Can you work these out from the model? Positions are in its coordinate system, mm. A direction names the side the tool comes from. Give positions to 0.01 mm unless a question says otherwise; leave off trailing zeros. Write each loop counter-clockwise with the first axis right and the second up, starting at its lowest first coordinate (ties: lowest second). Pieces come first, ordered by that corner, then holes.
```python
from build123d import *

# Parameters (mm, degrees)
SKETCH1_R           = 6
SKETCH1_R_2         = 4
BOSS_EXTRUDE1_DEPTH = 10
SKETCH2_R           = 6
BOSS_EXTRUDE2_DEPTH = 8
SKETCH3_R           = 5
SKETCH3_R_2         = 3
BOSS_EXTRUDE3_DEPTH = 10
SKETCH4_R           = 1.5
CUT_EXTRUDE1_DEPTH  = 10
SKETCH5_W           = 1.364712806
SKETCH5_H           = 6.528107361
CUT_EXTRUDE2_DEPTH  = 10
CHAMFER1_SIZE       = 1
SKETCH6_W           = 0.953233667
SKETCH6_H           = 4.701860643
CUT_EXTRUDE3_DEPTH  = 10


with BuildPart() as part:
    # Sketch1 → Boss-Extrude1 (new body)
    with BuildSketch(Plane(origin=(0, 0, 0), x_dir=(1, 0, 0), z_dir=(0, 1, 0))):
        with Locations(Location((0, 0, 0), (0, 0, 270))):
            Circle(SKETCH1_R)
        with Locations(Location((0, 0, 0), (0, 0, 270))):
            Circle(SKETCH1_R_2, mode=Mode.SUBTRACT)
    extrude(amount=BOSS_EXTRUDE1_DEPTH)

    # Sketch2 → Boss-Extrude2 (add)
    with BuildSketch(Plane(origin=(0, 10, 0), x_dir=(1, 0, 0), z_dir=(0, 1, 0))):
        with Locations(Location((0, 0, 0), (0, 0, 270))):
            Circle(SKETCH2_R)
    extrude(amount=BOSS_EXTRUDE2_DEPTH)

    # Sketch3 → Boss-Extrude3 (add)
    with BuildSketch(Plane(origin=(0, 18, 0), x_dir=(1, 0, 0), z_dir=(0, 1, 0))):
        with Locations(Location((0, 0, 0), (0, 0, 270))):
            Circle(SKETCH3_R)
        with Locations(Location((0, 0, 0), (0, 0, 270))):
            Circle(SKETCH3_R_2, mode=Mode.SUBTRACT)
    extrude(amount=BOSS_EXTRUDE3_DEPTH)

    # Sketch4 → Cut-Extrude1 (cut)
    with BuildSketch(Plane(origin=(0, 0, 0), x_dir=(0, 0, -1), z_dir=(1, 0, 0))):
        with Locations(Location((0, 5, 0), (0, 0, 180))):
            Circle(SKETCH4_R)
        with Locations(Location((0, 23, 0), (0, 0, 180))):
            Circle(SKETCH4_R)
    extrude(amount=CUT_EXTRUDE1_DEPTH, mode=Mode.SUBTRACT)

    # Sketch5 → Cut-Extrude2 (cut)
    with BuildSketch(Plane.XZ):
        with Locations((6.382356403, -0.325289304)):
            Rectangle(SKETCH5_W, SKETCH5_H)
    extrude(amount=-CUT_EXTRUDE2_DEPTH, mode=Mode.SUBTRACT)

    # Chamfer1
    # the kernel refuses this chamfer: 1 mm, written as the material it adds along each edge
    with BuildSketch(Plane(origin=(5.7, 10, -4.445182387), x_dir=(-0.02749587661058651, -0.9996219169112968, 0), z_dir=(0, 0, 1))) as chamfer1_piece_1_section:
        Polygon((CHAMFER1_SIZE * 0.999621916911, CHAMFER1_SIZE * 0.0274958766106), (-CHAMFER1_SIZE * 0.0274958766106, CHAMFER1_SIZE * 0.999621916911), (0, 0), align=None)
    chamfer1_piece_1 = extrude(amount=8.890364775, mode=Mode.PRIVATE)
    chamfer1_piece_1 = chamfer1_piece_1 & Plane(origin=(0, 9.556619027, 0), x_dir=(0, 0, 1), z_dir=(0, -1, 0)) * Cylinder(6, 22, mode=Mode.PRIVATE)
    add(chamfer1_piece_1)

    # Sketch6 → Cut-Extrude3 (cut)
    with BuildSketch(Plane(origin=(0, 28, 0), x_dir=(1, 0, 0), z_dir=(0, 1, 0))):
        with Locations((5.176616834, 0.047714229)):
            Rectangle(SKETCH6_W, SKETCH6_H)
    extrude(amount=-CUT_EXTRUDE3_DEPTH, mode=Mode.SUBTRACT)


solid = part.part
```
1) Please list where these lines run through material, in increasing order: L1, parallel to Y at x = 4.15, z = 0; L2, parallel to Y at x = 3.7, z = 0; L3, parallel to X at y = 25.5, z = 0.
Values follow:
L1: y = 0 to 3.5, 6.5 to 21.5, 24.5 to 28
L2: y = 10 to 21.5, 24.5 to 28
L3: x = -5 to -3, 3 to 4.7
2) Suppose I cut it at B-B on y = 23. Write out the boundary of the cut face in (x, z), plus the area to 3 significant figures.
Values follow:
outline: (2.6, -1.5) arc R3 cw (long way) to (2.6, 1.5) - (4.7, 1.5) - (4.7, 1.71) arc R5 ccw (long way) to (4.7, -1.71) - (4.7, -1.5) - close
area: 44.1 mm2
3) Suppose I cut it at C-C on y = 8.5. Write out the boundary of the cut face in (x, z).
Values follow:
outline: (5.7, -1.87) - (5.7, 1.87) arc R6 ccw (long way) to start; hole circle Ø8 at (0, 0)
4) For pin 1 Ø2.5 at (y, z) = (24.5, 0) entering from +X; pin 2 Ø0.5 at (x, z) = (5, 0) entering from +Y; pin 3 Ø3 at (x, y) = (-4.5, 25) entering from -Z, each with a flat end and sliding along its axis, tell me the tip position at first contact or that it passes through.
Values follow:
pin 1: stops at x = 4.7
pin 2: stops at y = 18
pin 3: stops at z = -4
5) Suppose I cut it at D-D on z = -3.5. Write out the boundary of the cut face in (x, y).
Values follow:
outline: (-4.87, 0) - (-1.94, 0) - (-1.94, 10) - (1.94, 10) - (1.94, 0) - (4.87, 0) - (4.87, 18) - (3.57, 18) - (3.57, 28) - (-3.57, 28) - (-3.57, 18) - (-4.87, 18) - close
6) For faces 1 (the face through (4.69, 4.55, 1.43)), 2 (the face through (-3.905, 4.93, -0.867)), 3 (the face through (0, 18, 0)), 4 (the face through (4.7, 24.2, 1.2)), 5 (the face through (5.7, 3, 0)), which set-ups out of +Z, -Z, +X, -X, +Y, -Y let a thin tool reach every point of the face, with its end or its side?
Values follow:
face 1: +X
face 2: -Y
face 3: +Y
face 4: +Z, -Z, +X, +Y
face 5: +Z, -Z, +X, -Y
7) If we mould it in two halves opening along Z, with no side actions, what happens to faces 6 (the face through (3.63, 22.55, 1.43)), 7 (the face through (-2.93, 22.93, -0.65)), 8 (the face through (-2.2, 28, -2.3))? For each: +Z half, -Z half, draft (parallel to the pull), parting line (faces both ways), or undercut.
Values follow:
face 6: undercut
face 7: undercut
face 8: draft
8) Suppose I cut it at A-A on z = 0. Write out the boundary of the cut face in (x, y).
Values follow:
outline: (-6, 0) - (-4, 0) - (-4, 10) - (4, 10) - (4, 6.5) - (5.7, 6.5) - (5.7, 9) - (6, 9.3) - (6, 18) - (4.7, 18) - (4.7, 21.5) - (3, 21.5) - (3, 18) - (-3, 18) - (-3, 28) - (-5, 28) - (-5, 18) - (-6, 18) - close; (3, 24.5) - (4.7, 24.5) - (4.7, 28) - (3, 28) - close; (4, 0) - (5.7, 0) - (5.7, 3.5) - (4, 3.5) - close
